Part model, mm, in its own coordinate system. A direction names the side the tool comes from. Coordinates: 2 decimals unless noted, no trailing zeros. Write each loop counter-clockwise with the first axis right and the second up, starting at its lowest first coordinate (ties: lowest second). Pieces come first, ordered by that corner, then holes. Notation, with made-up numbers: (-39, 71) -> (10, 71) arc R13 ccw to (10, 81) -> close; hole circle Ø4 at (59, -21.5). An arc over 180 degrees is marked (long way). Write item = value, one per line.
from build123d import *

# Parameters (mm, degrees)
CUT_EXTRUDE_1_DEPTH      = 20.514609912
CUT_EXTRUDE_1_DEPTH_BACK = 20.514609912
SKETCH_2_W               = 2.289640131
SKETCH_2_H               = 2


with BuildPart() as part:
    # 草图1 → 旋转1 (revolve)
    with BuildSketch(Plane.XY, mode=Mode.PRIVATE) as revolve_1_sk:
        Polygon((0, 0), (0, 7.9), (0.75, 7.9), (4.65, 4), (16, 4), (16, 0), align=None)
    revolve(revolve_1_sk.sketch.rotate(Axis((-3.228581577, 0, 0), (1, 0, 0)), 90), axis=Axis((-3.228581577, 0, 0), (1, 0, 0)))

    # 草图2 → 切除-拉伸1 (cut, two sides: drawn at the far end of the back side and taken through both)
    with BuildSketch(Plane.XY.offset(-CUT_EXTRUDE_1_DEPTH_BACK)):
        with Locations((0.655179935, 0)):
            Rectangle(SKETCH_2_W, SKETCH_2_H)
    extrude(amount=CUT_EXTRUDE_1_DEPTH + CUT_EXTRUDE_1_DEPTH_BACK, mode=Mode.SUBTRACT)


solid = part.part
Q1. Saw through at C-C on x = 8.75. Give the cut face in (y, z), and give its area (3 significant figures).
Model answer:
outline = circle Ø8 at (0, 0)
area = 50.3 mm²
Q2. Probe line 1 (Y direction, x = 1.75, z = 1); line 2 (Y direction, x = 7.25, z = 3.5); line 3 (Y direction, x = 13.25, z = 1.5). List the from-to ranges inside material, lowest first. Write a range as from..to.
Model answer:
line_1 = -6.83..-1, 1..6.83
line_2 = -1.94..1.94
line_3 = -3.71..3.71
Q3. Saw through at A-A on z = 0. Give the cut face in (x, y).
Model answer:
outline = (0, -7.9) -> (0.75, -7.9) -> (4.65, -4) -> (16, -4) -> (16, 4) -> (4.65, 4) -> (0.75, 7.9) -> (0, 7.9) -> (0, 1) -> (1.8, 1) -> (1.8, -1) -> (0, -1) -> close
Q4. Mould opens along Y. For faces 1 (the face through (16, 0, 0)), 2 (the face through (1.8, 0, 0)), 3 (the face through (1, -1, 0)), 4 (the face through (4.461, -1.258, 3.996)) say: released by +Y, released by -Y, zero draft, split by the parting line, or undercut.
Model answer:
face_1 = zero draft
face_2 = undercut
face_3 = undercut
face_4 = split by the parting line
Q5. Saw through at B-B on y = 0. Give the cut face in (x, z).
Model answer:
outline = (1.8, -6.85) -> (4.65, -4) -> (16, -4) -> (16, 4) -> (4.65, 4) -> (1.8, 6.85) -> close
Q6. Pin check, flat tips, straight feed: pin 1 (4 mm diameter, centred on x = 10.5, y = -4.5, fed in from -Z); pin 2 (3 mm diameter, centred on x = 10.5, z = 3.5, fed in from +Y); pin 3 (0.9 mm diameter, centred on x = 0.5, z = 1, fed in from +Y). Stop position of each tip, or through.
Model answer:
pin_1 = -3.12
pin_2 = 3.46
pin_3 = 7.88
Q7. Which spindle directions (+Z, -Z, +X, -X, +Y, -Y) get a long thin tool onto all of the face, cutting with end or side? Do faces 5 (the face through (0.38, 7.9, -0.16)), 6 (the face through (1, 1, 0)), 7 (the face through (10.404, 3.905, -0.867)). Say none if no direction does.
Model answer:
face_5 = +X, -X, +Y
face_6 = +Z, -Z, -X
face_7 = +X
